from build123d import *

# Parameters (mm, degrees)
ESQUISSE8_W        = 140
ESQUISSE8_H        = 80
BOSS_EXTRU_7_DEPTH = 8


with BuildPart() as part:
    # Esquisse8 → Boss.-Extru.7 (new body)
    with BuildSketch(Plane.XY):
        with Locations((-153.601186705, 56.489400981)):
            Rectangle(ESQUISSE8_W, ESQUISSE8_H)
        with BuildLine():
            Line((-193.601186705, 68.887436176), (-113.601186705, 68.887436176))
            ThreePointArc((-113.601186705, 68.887436176), (-101.203151511, 56.489400981), (-113.601186705, 44.091365787))
            Line((-113.601186705, 44.091365787), (-193.601186705, 44.091365787))
            ThreePointArc((-193.601186705, 44.091365787), (-205.9992219, 56.489400981), (-193.601186705, 68.887436176))
        make_face(mode=Mode.SUBTRACT)
        with BuildLine():
            Line((-187.470030447, 38.922719402), (-137.470030447, 38.922719402))
            ThreePointArc((-137.470030447, 38.922719402), (-131.485282002, 32.937970956), (-137.470030447, 26.953222511))
            Line((-137.470030447, 26.953222511), (-187.470030447, 26.953222511))
            ThreePointArc((-187.470030447, 26.953222511), (-193.454778893, 32.937970956), (-187.470030447, 38.922719402))
        make_face(mode=Mode.SUBTRACT)
    extrude(amount=BOSS_EXTRU_7_DEPTH)


solid = part.part
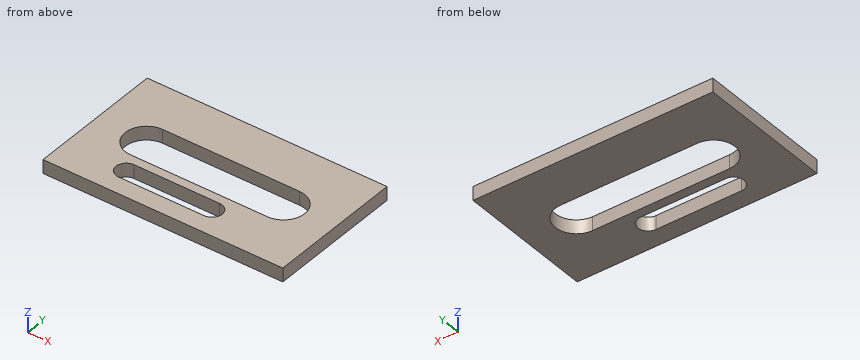
Verification items for the finished model (mm, model axes). Coordinates: 2 decimals unless noted, no trailing zeros. Write each loop counter-clockwise with the first axis right and the second up, starting at its lowest first coordinate (ties: lowest second). Pieces come first, ordered by that corner, then holes. Notation, with made-up numbers: (-22.75, -37.75) - (5.25, -37.75) arc R29 cw to (5.25, -17.75) - close; hole circle Ø5 at (69.25, -15). An arc over 180 degrees is marked (long way). Answer as a JSON object with one key per item and string values.
(1) Cross-section at A-A on x = -176. Record the cut outline in (y, z), plus the area to 3 significant figures.
Report:
{"outline": "(16.49, 0) - (26.95, 0) - (26.95, 8) - (16.49, 8) - close; (38.92, 0) - (44.09, 0) - (44.09, 8) - (38.92, 8) - close; (68.89, 0) - (96.49, 0) - (96.49, 8) - (68.89, 8) - close", "area": "346 mm^2"}
(2) Gauge pin test, flat end, axial feed: pin 1 Ø2 at (x, y) = (-129, 70.5) entering from -Z. Record the tip position at first contact, or that the pin passes through.
Report:
{"pin 1": "z = 0"}
(3) Cross-section at C-C on y = 67.5. Record the cut outline in (x, z), plus the area to 3 significant figures.
Report:
{"outline": "(-223.6, 0) - (-199.3, 0) - (-199.3, 8) - (-223.6, 8) - close; (-107.9, 0) - (-83.6, 0) - (-83.6, 8) - (-107.9, 8) - close", "area": "389 mm^2"}
(4) Cross-section at B-B on z = 3. Record the cut outline in (x, y).
Report:
{"outline": "(-223.6, 16.49) - (-83.6, 16.49) - (-83.6, 96.49) - (-223.6, 96.49) - close; hole (-193.6, 44.09) - (-113.6, 44.09) arc R12.4 ccw to (-113.6, 68.89) - (-193.6, 68.89) arc R12.4 ccw to start; hole (-187.47, 26.95) - (-137.47, 26.95) arc R5.98 ccw to (-137.47, 38.92) - (-187.47, 38.92) arc R5.98 ccw to start"}
(5) Thickness scan on line 1 along Y through (x, z) = (-183.5, 6.5); line 2 along X through (y, z) = (32.5, 3); line 3 along Y through (x, z) = (-114, 4). Record the ranges inside material, lowest first.
Report:
{"line 1": "16.49 to 26.95, 38.92 to 44.09, 68.89 to 96.49", "line 2": "-223.6 to -193.44, -131.5 to -83.6", "line 3": "16.49 to 44.09, 68.89 to 96.49"}
(6) Cross-section at D-D on x = -133.5. Record the cut outline in (y, z), plus the area to 3 significant figures.
Report:
{"outline": "(16.49, 0) - (28.46, 0) - (28.46, 8) - (16.49, 8) - close; (37.42, 0) - (44.09, 0) - (44.09, 8) - (37.42, 8) - close; (68.89, 0) - (96.49, 0) - (96.49, 8) - (68.89, 8) - close", "area": "370 mm^2"}
